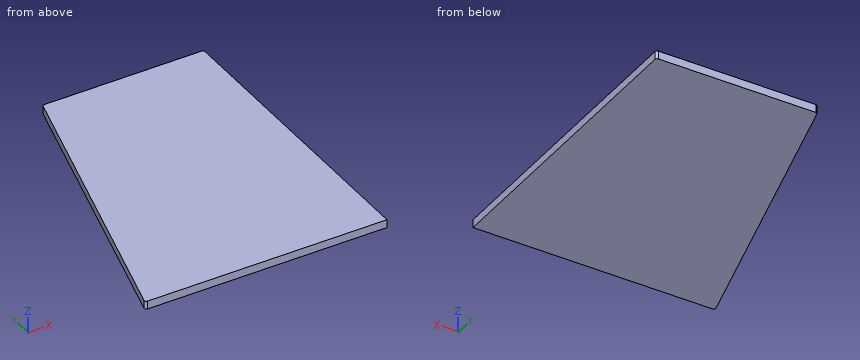
Autodesk Inventor part; units mm, degrees
ref_plane "YZ Plane" through (0, 0, 0) normal (1, 0, 0) x (0, 1, 0)
ref_plane "XZ Plane" through (0, 0, 0) normal (0, 1, 0) x (-1, 0, 0)
ref_plane "XY Plane" through (0, 0, 0) normal (0, 0, 1) x (1, 0, 0)
sketch "Sketch1" plane through (0, 0, 0) normal (0, 0, 1) x (1, 0, 0)
  line L0 (-160, 0) -> (0, 0)
  line L1 (-160, -300) -> (-160, 0) construction
  line L2 (-160, 0) -> (-240.3848, -300)
  line L3 (-240.3848, -300) -> (-160, -300)
  line L4 (0, 0) -> (-80.3848, -300) construction
  line L5 (0, 0) -> (160, 0)
  line L6 (0, 0) -> (0, -300)
  line L7 (0, -300) -> (-160, -300)
  dimension "d2" = 15
  dimension "d29" = 160
  dimension "d40" = 300
  dimension "d41" = 15
extrude "Plate1" add sketch "Sketch1" along normal blind 8
fillet "Corner Round1" radius 2 3 edges at (-240.3848, -300, 4) (0, 0, 4) (-160, 0, 4)
equation "\"d3\" = Thickness"
equation "\"BendRadius\" = Thickness"
equation "\"BendReliefWidth\" = Thickness"
equation "\"BendReliefDepth\" = 0.5 * Thickness"
equation "\"CornerReliefSize\" = 4 * Thickness"
equation "\"MinimumRemnant\" = 2 * Thickness"
equation "\"TransitionRadius\" = BendRadius"
equation "\"JacobiRadiusSize\" = BendRadius"
equation "\"GapSize\" = Thickness"
properties part number "Сrane plate 4"
Geometry: final body of the model. Coordinates: model frame, mm. Coordinates: 2 decimals unless noted, no trailing zeros. Order: outer loops, then holes, each group sorted by start corner. A loop starts at its lowest first (then second) coordinate and runs counter-clockwise, first axis right, second up. Notation, with made-up numbers: M 50.25,88.25 L 99.25,88.25 A28 ccw 99.25,127.25 Z; hole C 35.25,23 d2. An arc over 180 degrees is marked long. Answer as CSV lines item,"result".
Q1. Section B-B on y = -63. Return the cut outline in (x, z).
Answers:
outline,"M -176.88,0 L 0,0 L 0,8 L -176.88,8 Z"
Q2. Section C-C on x = -214. Return the cut outline in (y, z), and give its area (3 significant figures).
Answers:
outline,"M -300,0 L -201.53,0 L -201.53,8 L -300,8 Z"
area,"788 mm^2"
Q3. First-contact query: P1, Ø4, axis at x = -179.5, y = -223.5, coming from the -Z side. Flat tip, straight axial feed; report the tip coordinate or a pass-through.
Answers:
P1,"stops at z = 0"
Q4. Line query: probe 1 along X at (y, z) = (-59.5, 2.75); probe 2 along X at (y, z) = (-216, 7.5). Output: solid intervals per line, ascending. Write a range as [from, to].
Answers:
probe 1,"x = [-175.94, 0]"
probe 2,"x = [-217.88, 0]"
Q5. Section A-A on z = 1.5. Return the cut outline in (x, y).
Answers:
outline,"M -239.71,-297.48 A2 ccw -237.78,-300 L 0,-300 L 0,-2 A2 ccw -2,0 L -158.47,0 A2 ccw -160.4,-1.48 Z"
